For this review, take the finished solid that the model builds, in its own axes (mm). A direction names the side the tool comes from. Round coordinates to 2 decimals unless told otherwise and drop trailing zeros. Loops run counter-clockwise (first coordinate to the right, second up) from the corner with the lowest first, then second, coordinate; pieces in that order, holes last. Notation, with made-up numbers: (61.5, 84.25) -> (65.5, 84.25) arc R18 cw to (65.5, 110.25) -> close; hole circle Ø4 at (68.25, -11). An arc over 180 degrees is marked (long way). Write each question's results on one line, items separated by ' | '.
Autodesk Inventor part; units mm, degrees
ref_plane "YZ Plane" through (0, 0, 0) normal (1, 0, 0) x (0, 1, 0)
ref_plane "XZ Plane" through (0, 0, 0) normal (0, 1, 0) x (-1, 0, 0)
ref_plane "XY Plane" through (0, 0, 0) normal (0, 0, 1) x (1, 0, 0)
sketch "Sketch1" plane through (0, 0, 0) normal (0, 0, 1) x (1, 0, 0)
  line L0 (-22.5, 0) -> (22.5, 0)
  line L1 (22.5, 0) -> (22.5, 5)
  line L2 (-22.5, 0) -> (-22.5, 5)
  line L3 (-22.5, 5) -> (-9.5, 5)
  line L4 (22.5, 5) -> (9.5, 5)
  line L5 (-9.5, 5) -> (-9.5, 10)
  line L6 (9.5, 5) -> (9.5, 10)
  arc A0 (4, 18.6042) -> (-4, 18.6042) centre (0, 27) ccw
  line L7 (4, 18.6042) -> (8.9676, 10)
  line L8 (-4, 18.6042) -> (-8.9676, 10)
  line L9 (-9.5, 10) -> (9.5, 10) construction
  line L10 (-8.9676, 10) -> (-9.5, 10) construction
  line L11 (-8.9676, 10) -> (-9.5, 10)
  line L12 (8.9676, 10) -> (9.5, 10)
  line L13 (-11.4601, 5) -> (-11.4601, 0) construction
  line L14 (-16.9601, 5) -> (-16.9601, 0) construction
  line L15 (13.0399, 5) -> (13.0399, 0) construction
  line L16 (18.5399, 5) -> (18.5399, 0) construction
  arc A1 (-4, 18.6042) -> (4, 18.6042) centre (0, 27) ccw construction
  point P0 (0, 0)
  point P1 (0, 0)
  point P2 (0, 17.7)
  point P3 (15.7899, 5)
  point P4 (-14.2101, 5)
  dimension "B" = 45
  dimension "t" = 5
  dimension "d2" = 5
  dimension "dimensionf" = 19
  dimension "d4" = 13
  dimension "Y" = 10
  dimension "d6" = 5
  dimension "d" = 18.6
  dimension "e" = 22.5
  dimension "dimensionH" = 17.7
  dimension "dimensionh" = 27
  dimension "x" = 8
  dimension "d16" = 4
  dimension "dimensionc" = 30
  dimension "d21" = 6.7101
  dimension "s1" = 5.5
  dimension "d23" = 5.5
  dimension "d24" = 2.75
  dimension "d25" = 2.75
extrude "Extrusion1" add sketch "Sketch1" along normal blind 500
equation "\"d2\" = t"
properties part number "sbr20_500mm"
1. Consider section A-A (z = 94). State the section outline as (x, y) points.
Values found:
outline: (-22.5, 0) -> (22.5, 0) -> (22.5, 5) -> (9.5, 5) -> (9.5, 10) -> (8.97, 10) -> (4, 18.6) arc R9.3 ccw (long way) to (-4, 18.6) -> (-8.97, 10) -> (-9.5, 10) -> (-9.5, 5) -> (-22.5, 5) -> close
2. For pin 1 (5 mm diameter, centred on y = 31.5, z = 380.5, fed in from -X); pin 2 (14.5 mm diameter, centred on x = 13, z = 171, fed in from +Y); pin 3 (2.5 mm diameter, centred on y = 7.5, z = 133, fed in from +X), all flat-tipped, find the tip position at first contact; note any pin that passes through.
Values found:
pin 1: stops at x = -9.08 | pin 2: stops at y = 34.31 | pin 3: stops at x = 9.5
3. Draft analysis for pull direction Y (two halves, no side actions). For faces 4 (the face through (0, 14, 500)), 5 (the face through (6.45, 14.36, 246.5)), 6 (the face through (-0.351, 36.293, 246.5)), 7 (the face through (-16, 5, 246)), state which applies: released by +Y, released by -Y, zero draft, split by the parting line, or undercut.
Values found:
face 4: zero draft | face 5: undercut | face 6: undercut | face 7: released by +Y
4. Tool access review of faces 1 (the face through (-6.45, 14.36, 246.5)), 2 (the face through (0, 0, 246)), 3 (the face through (16, 5, 246)): name each direction out of +Z, -Z, +X, -X, +Y, -Y from which nothing blocks a thin tool from reaching the whole face with its end or side.
Values found:
face 1: +Z, -Z, -X | face 2: +Z, -Z, +X, -X, -Y | face 3: +Z, -Z, +X, +Y
5. Consider section B-B (y = 27). State the section outline as (x, z) points.
Values found:
outline: (-9.3, 0) -> (9.3, 0) -> (9.3, 500) -> (-9.3, 500) -> close
6. Consider section C-C (x = 18). State the section outline as (y, z) points.
Values found:
outline: (0, 0) -> (5, 0) -> (5, 500) -> (0, 500) -> close
7. To check wall thickness, follow probe 1 along X at (y, z) = (9, 208.5); probe 2 along X at (y, z) = (27, 150.5); probe 3 along Y at (x, z) = (-15, 405.5). State the ranges of each line that lie inside material, in increasing order.
Values found:
probe 1: x = -9.5 to 9.5 | probe 2: x = -9.3 to 9.3 | probe 3: y = 0 to 5
